The figure shows three views and two pictorial views of one solid part (mm, origin at its lowest corner). Answer the questions. A direction names the side the tool comes from. Give positions to 0.01 mm unless a question says otherwise; leave off trailing zeros. Loops run counter-clockwise (first coordinate to the right, second up) from the corner with the lowest first, then second, coordinate; pieces in that order, holes last. Notation, with made-up numbers: (77, 13) -> (82, 13) arc R27 cw to (82, 32) -> close; hole circle Ø1 at (69, -33.5). An arc over 180 degrees is marked (long way). Answer as CSV lines item,"result". Start each with the question number.
1. Flat-ended cylindrical pins translate along their axes: pin 1 Ø10 at (x, z) = (68, 33) entering from +Y; pin 2 Ø3 at (y, z) = (16, 9.5) entering from -X; pin 3 Ø2 at (x, y) = (32, 36.5) entering from +Z; pin 4 Ø5 at (x, z) = (81.5, 49.5) entering from +Y. Find the tip coordinate at first contact, or state that the pin passes through.
2. Find the intervals of material crossed by line 1 along X through (y, z) = (20, 48); line 2 along Z through (x, y) = (80, 26.25); line 3 along X through (y, z) = (52.5, 4), in increasing order.
3. Find section C-C, the plane z = 7. Give the vertices of the cut face in (x, y).
4. Find section B-B, the plane x = 20. Give the vertices of the cut face in (y, z), and give its area (3 significant figures).
5. Find section D-D, the plane y = 52.5. Give the vertices of the cut face in (x, z).
6. A tool of negligible diameter and unlimited length cuts with its end or side. For the marked faces 4, 5, 6, 7 and 8, from which of +Z, -Z, +X, -X, +Y, -Y can it reach the whole face along a straight path? Write none if from no direction.
7. Determine the mould class of the marked faces 1, 2 and 3 for opening direction X: +X half, -X half, draft (parallel to the pull), parting line (faces both ways), or undercut.
8. Find section A-A, the plane y = 44.45. Give the vertices of the cut face in (x, z), and give its area (3 significant figures).
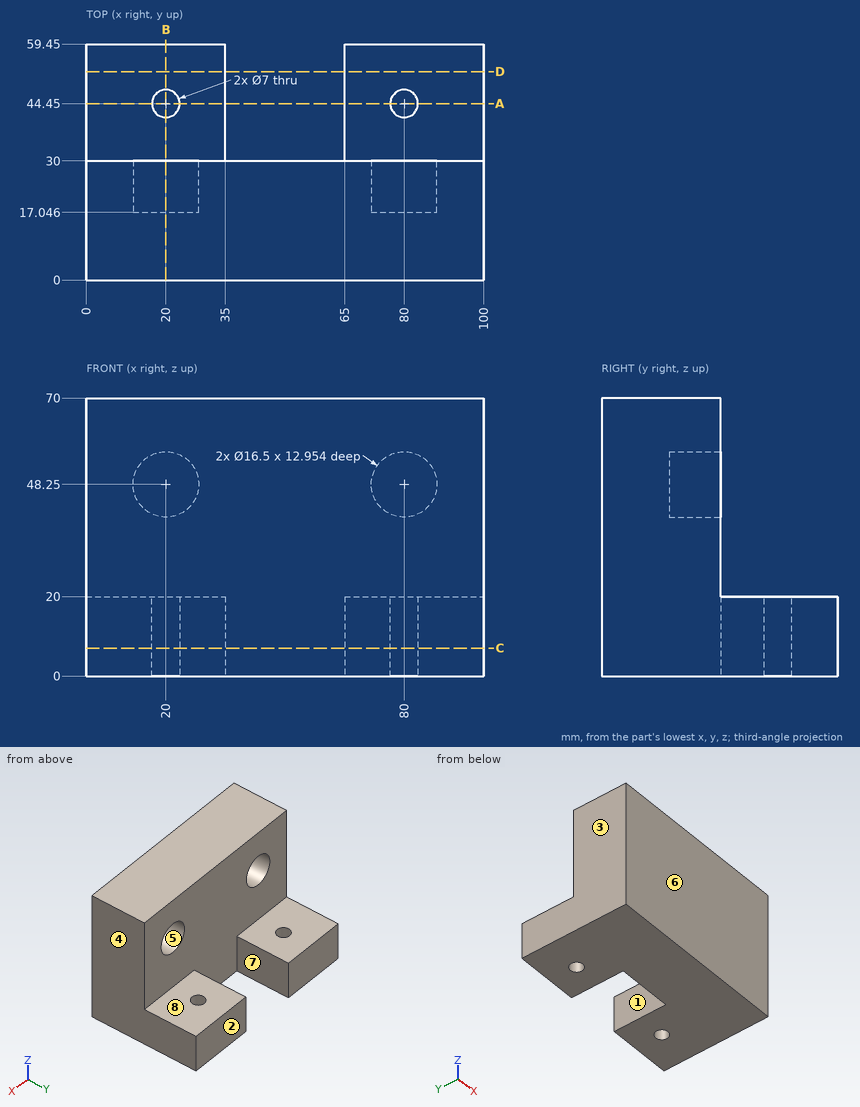
Resolved:
1,pin 1,"stops at y = 30"
1,pin 2,"stops at x = 0"
1,pin 3,"stops at z = 20"
1,pin 4,"stops at y = 17.05"
2,line 1,"x = 0 to 11.75, 28.25 to 71.75, 88.25 to 100"
2,line 2,"z = 0 to 40, 56.5 to 70"
2,line 3,"x = 0 to 35, 65 to 100"
3,outline,"(0, 0) -> (100, 0) -> (100, 59.45) -> (65, 59.45) -> (65, 30) -> (35, 30) -> (35, 59.45) -> (0, 59.45) -> close; hole circle Ø7 at (20, 44.45); hole circle Ø7 at (80, 44.45)"
4,outline,"(0, 0) -> (40.95, 0) -> (40.95, 20) -> (30, 20) -> (30, 40) -> (17.05, 40) -> (17.05, 56.5) -> (30, 56.5) -> (30, 70) -> (0, 70) -> close; (47.95, 0) -> (59.45, 0) -> (59.45, 20) -> (47.95, 20) -> close"
4,area,"2,340 mm^2"
5,outline,"(0, 0) -> (35, 0) -> (35, 20) -> (0, 20) -> close; (65, 0) -> (100, 0) -> (100, 20) -> (65, 20) -> close"
6,face 4,"+Z, -Z, +X, +Y, -Y"
6,face 5,"+Y"
6,face 6,"+Z, -Z, +X, -X, -Y"
6,face 7,"+Z, -Z, +Y"
6,face 8,"+Z, +X, -X, +Y"
7,face 1,"undercut"
7,face 2,"draft"
7,face 3,"-X half"
8,outline,"(0, 0) -> (16.5, 0) -> (16.5, 20) -> (0, 20) -> close; (23.5, 0) -> (35, 0) -> (35, 20) -> (23.5, 20) -> close; (65, 0) -> (76.5, 0) -> (76.5, 20) -> (65, 20) -> close; (83.5, 0) -> (100, 0) -> (100, 20) -> (83.5, 20) -> close"
8,area,"1,120 mm^2"
